from build123d import *

# Parameters (mm, degrees)
CYLINDER001_R          = 2.5
CYLINDER001_DEPTH      = 20
CYLINDER002_R          = 2.5
CYLINDER002_DEPTH      = 20
CYLINDER004_R          = 2.5
CYLINDER004_DEPTH      = 20
CYLINDER005_R          = 2.5
CYLINDER005_DEPTH      = 20
CYLINDER003_R          = 2.5
CYLINDER003_DEPTH      = 20
CYLINDER_R             = 2.5
CYLINDER_DEPTH         = 20
BOX004_W               = 50
BOX004_H               = 8
BOX004_DEPTH           = 90
CHAMFER_SIZE           = 4
CHAMFER001_SIZE        = 2
BOX002_W               = 15
BOX002_H               = 177
BOX002_DEPTH           = 100
BOX003_W               = 15
BOX003_H               = 125
BOX003_DEPTH           = 18
BOX003_PLACEMENT_ANGLE = 28
BOX001_W               = 15
BOX001_H               = 163
BOX001_DEPTH           = 100
BOX_W                  = 15
BOX_H                  = 187
BOX_DEPTH              = 100
CHAMFER002_SIZE        = 4


with BuildPart() as cylinder001:
    # Cylinder001 → Cylinder001 (new body)
    with BuildSketch(Plane(origin=(-8.5, 14, 15), x_dir=(1, 0, 0), z_dir=(0, -1, 0))):
        Circle(CYLINDER001_R)
    extrude(amount=CYLINDER001_DEPTH)


with BuildPart() as cylinder002:
    # Cylinder002 → Cylinder002 (new body)
    with BuildSketch(Plane(origin=(23.55, 14, 45), x_dir=(1, 0, 0), z_dir=(0, -1, 0))):
        Circle(CYLINDER002_R)
    extrude(amount=CYLINDER002_DEPTH)


with BuildPart() as cylinder004:
    # Cylinder004 → Cylinder004 (new body)
    with BuildSketch(Plane(origin=(23.55, 14, 75), x_dir=(1, 0, 0), z_dir=(0, -1, 0))):
        Circle(CYLINDER004_R)
    extrude(amount=CYLINDER004_DEPTH)


with BuildPart() as cylinder005:
    # Cylinder005 → Cylinder005 (new body)
    with BuildSketch(Plane(origin=(-8.5, 14, 75), x_dir=(1, 0, 0), z_dir=(0, -1, 0))):
        Circle(CYLINDER005_R)
    extrude(amount=CYLINDER005_DEPTH)


with BuildPart() as cylinder003:
    # Cylinder003 → Cylinder003 (new body)
    with BuildSketch(Plane(origin=(-8.5, 14, 45), x_dir=(1, 0, 0), z_dir=(0, -1, 0))):
        Circle(CYLINDER003_R)
    extrude(amount=CYLINDER003_DEPTH)


with BuildPart() as compound:
    # Cylinder → Cylinder (new body)
    with BuildSketch(Plane(origin=(23.55, 14, 15), x_dir=(1, 0, 0), z_dir=(0, -1, 0))):
        Circle(CYLINDER_R)
    extrude(amount=CYLINDER_DEPTH)

    # Compound: union Cylinder001, Cylinder002, Cylinder004, Cylinder005, Cylinder003
    add(cylinder001.part)
    add(cylinder002.part)
    add(cylinder004.part)
    add(cylinder005.part)
    add(cylinder003.part)


with BuildPart() as backplate:
    # Box004 → Box004 (new body)
    with BuildSketch(Plane(origin=(-17.5, 0, 0), x_dir=(1, 0, 0), z_dir=(0, 0, 1))):
        with Locations((25, 4)):
            Rectangle(BOX004_W, BOX004_H)
    extrude(amount=BOX004_DEPTH)

    # Chamfer
    chamfer_edges = [backplate.edges().sort_by_distance(p)[0] for p in [
        (-17.5, 4, 90),
        (-17.5, 4, 0),
        (32.5, 4, 90),
        (32.5, 4, 0),
    ]]
    chamfer(chamfer_edges, length=CHAMFER_SIZE)

    # Cut001: cut Compound
    add(compound.part, mode=Mode.SUBTRACT)

    # Chamfer001
    chamfer001_edges = [backplate.edges().sort_by_distance(p)[0] for p in [
        (21.05, 8, 45),
        (-11, 8, 45),
        (-11, 8, 75),
        (21.05, 8, 75),
        (21.05, 8, 15),
        (-11, 8, 15),
    ]]
    chamfer(chamfer001_edges, length=CHAMFER001_SIZE)


with BuildPart() as cube002:
    # Box002 → Box002 (new body)
    with BuildSketch(Plane(origin=(0, 5, 90), x_dir=(1, 0, 0), z_dir=(0, 0, 1))):
        with Locations((7.5, 88.5)):
            Rectangle(BOX002_W, BOX002_H)
    extrude(amount=BOX002_DEPTH)


with BuildPart() as cube003:
    # Box003 → Box003 (new body)
    with BuildSketch(Plane.XY):
        with Locations((7.5, 62.5)):
            Rectangle(BOX003_W, BOX003_H)
    extrude(amount=BOX003_DEPTH)


with BuildPart() as cube003_1:
    # Box003 placement: moved
    add(cube003.part.moved(Location((0, 20, 11.25))).rotate(Axis((0, 20, 11.25), (1, 0, 0)), BOX003_PLACEMENT_ANGLE))


with BuildPart() as cube001:
    # Box001 → Box001 (new body)
    with BuildSketch(Plane(origin=(0, 34, -30), x_dir=(1, 0, 0), z_dir=(0, 0, 1))):
        with Locations((7.5, 81.5)):
            Rectangle(BOX001_W, BOX001_H)
    extrude(amount=BOX001_DEPTH)


with BuildPart() as final:
    # Box → Box (new body)
    with BuildSketch(Plane.XY):
        with Locations((7.5, 93.5)):
            Rectangle(BOX_W, BOX_H)
    extrude(amount=BOX_DEPTH)

    # Cut: cut Cube001
    add(cube001.part, mode=Mode.SUBTRACT)

    # Fusion: union Cube003
    add(cube003_1.part)

    # Cut002: cut Cube002
    add(cube002.part, mode=Mode.SUBTRACT)

    # Chamfer002
    chamfer002_edges = [final.edges().sort_by_distance(p)[0] for p in [
        (7.5, 187, 70),
        (7.5, 34, 0),
    ]]
    chamfer(chamfer002_edges, length=CHAMFER002_SIZE)

    # Fusion001: union Backplate
    add(backplate.part)


solid = final.part
Input: part model. Units: mm. Frame: model coordinates. A direction names the side the tool comes from. Coordinates: 2 decimals unless noted, no trailing zeros. Loops run counter-clockwise (first coordinate to the right, second up) from the corner with the lowest first, then second, coordinate; pieces in that order, holes last. Notation, with made-up numbers: (53, 16) -> (79, 16) arc R19 ccw to (79, 47) -> close; hole circle Ø7 at (47, -3). An arc over 180 degrees is marked (long way). Write item = value, one per line. Start each with the question number.
Item 1: Material intervals for line 1 (Z direction, x = 23.55, y = 1.6); line 2 (Z direction, x = 23, y = 4); line 3 (X direction, y = 3.8, z = 45), sorted ascending.
Item 2: Reachability of faces 5 (the face through (7, 63, 70)), 6 (the face through (15, 76, 57)), 7 (the face through (7, 5, 95)), 8 (the face through (0, 76, 60)), 9 (the face through (7, 187, 87)) from +Z, -Z, +X, -X, +Y, -Y: full face, straight path, thin tool, end or side. Return the list, or none.
Item 3: Cut plane C-C, the plane x = 12. Return loops of the section in (y, z).
Item 4: Mould query, pull axis X, two halves, no side actions, for faces 1 (the face through (7, 182, 95)), 2 (the face through (24.7, 3.04, 72.78)), 3 (the face through (-15.5, 3.9, 88)), 4 (the face through (23.01, 3.04, 12.56)). Classes: pulls with the +X half, pulls with the -X half, needs draft (parallel to the pull), parting line crosses it, or undercut.
Item 5: First-contact query: P1, Ø5, axis at x = 9.5, z = 94.5, coming from the -Y side; P2, Ø12, axis at x = 11, y = 169.5, coming from the -Z side; P3, Ø10, axis at x = 20.5, y = 155.5, coming from the +Z side; P4, Ø4, axis at y = 38.5, z = 81, coming from the +X side. Flat tips, straight axial feed; report the tip coordinate or a pass-through.
Item 6: Cut plane A-A, the plane x = 23.55. Return loops of the section in (y, z).
Item 7: Cut plane B-B, the plane z = 45. Return loops of the section in (x, y).
Item 8: Cut plane D-D, the plane y = 82. Return loops of the section in (x, z).
Ans:
q1.line_1 = 0 to 12.5, 17.5 to 42.5, 47.5 to 72.5, 77.5 to 90
q1.line_2 = 0 to 12.56, 17.44 to 42.56, 47.44 to 72.56, 77.44 to 90
q1.line_3 = -17.5 to -11, -6 to 21.05, 26.05 to 32.5
q2.face_5 = +X, -X
q2.face_6 = +Z, -Z, +X, +Y
q2.face_7 = +Z, +X, -X
q2.face_8 = +Z, -Z, -X, +Y
q2.face_9 = +Z, -Z, +X, -X, +Y
q3.outline = (0, 0) -> (30, 0) -> (34, 4) -> (34, 18.69) -> (130.37, 69.93) -> (130.33, 70) -> (183, 70) -> (187, 74) -> (187, 100) -> (182, 100) -> (182, 90) -> (5, 90) -> (5, 100) -> (0, 100) -> close; hole (34, 39.08) -> (92.15, 70) -> (34, 70) -> close
q4.face_1 = needs draft
q4.face_2 = undercut
q4.face_3 = pulls with the -X half
q4.face_4 = undercut
q5.P1 = 0
q5.P2 = 70
q5.P3 = through
q5.P4 = 15
q6.outline = (0, 0) -> (8, 0) -> (8, 10.5) -> (6, 12.5) -> (0, 12.5) -> close; (0, 17.5) -> (6, 17.5) -> (8, 19.5) -> (8, 40.5) -> (6, 42.5) -> (0, 42.5) -> close; (0, 47.5) -> (6, 47.5) -> (8, 49.5) -> (8, 70.5) -> (6, 72.5) -> (0, 72.5) -> close; (0, 77.5) -> (6, 77.5) -> (8, 79.5) -> (8, 90) -> (0, 90) -> close
q7.outline = (-17.5, 0) -> (-11, 0) -> (-11, 6) -> (-13, 8) -> (-17.5, 8) -> close; (-6, 0) -> (21.05, 0) -> (21.05, 6) -> (19.05, 8) -> (15, 8) -> (15, 34) -> (0, 34) -> (0, 8) -> (-4, 8) -> (-6, 6) -> close; (0, 45.13) -> (15, 45.13) -> (15, 83.47) -> (0, 83.47) -> close; (26.05, 0) -> (32.5, 0) -> (32.5, 8) -> (28.05, 8) -> (26.05, 6) -> close
q8.outline = (0, 44.22) -> (15, 44.22) -> (15, 64.6) -> (0, 64.6) -> close; (0, 70) -> (15, 70) -> (15, 90) -> (0, 90) -> close
